```python
from build123d import *

# Parameters (mm, degrees)
SKETCH_1_R          = 14
EXTRUDE_1_DEPTH     = 4.5
CHAMFER_1_SIZE      = 2.25
SKETCH_2_R          = 10.75
EXTRUDE_2_DEPTH     = 25
CUT_EXTRUDE_START   = -25
CUT_EXTRUDE_1_DEPTH = 25
SKETCH_4_R          = 6
CUT_EXTRUDE_2_DEPTH = 5
EXTRUDE_3_DEPTH     = 5
CHAMFER_2_SIZE      = 0.5
EXTRUDE_4_DEPTH     = 3
SKETCH_7_R          = 2.5
CUT_EXTRUDE_3_DEPTH = 10


with BuildPart() as part:
    # 草图1 → 凸台-拉伸1 (new body)
    with BuildSketch(Plane(origin=(0, 0, 0), x_dir=(1, 0, 0), z_dir=(0, 1, 0))):
        with Locations(Location((0, 0, 0), (0, 0, 270))):
            Circle(SKETCH_1_R)
    extrude(amount=EXTRUDE_1_DEPTH)

    # 倒角1
    chamfer_1_edges = [part.edges().sort_by_distance(p)[0] for p in [
        (0, 4.5, -14),
    ]]
    chamfer(chamfer_1_edges, length=CHAMFER_1_SIZE)

    # 草图2 → 凸台-拉伸2 (add)
    with BuildSketch(Plane.XZ):
        with Locations(Location((0, 0, 0), (0, 0, 90))):
            Circle(SKETCH_2_R)
    extrude(amount=EXTRUDE_2_DEPTH)

    # 草图3 → 切除-拉伸1 (cut)
    with BuildSketch(Plane.XZ.offset(25).offset(CUT_EXTRUDE_START)):
        with BuildLine():
            Line((-3.94493346, -10), (3.94493346, -10))
            ThreePointArc((3.94493346, -10), (0, -10.75), (-3.94493346, -10))
        make_face()
        with BuildLine():
            Line((-3.94493346, 10), (3.94493346, 10))
            ThreePointArc((3.94493346, 10), (0, 10.75), (-3.94493346, 10))
        make_face()
    extrude(amount=CUT_EXTRUDE_1_DEPTH, mode=Mode.SUBTRACT)

    # 草图4 → 切除-拉伸2 (cut)
    with BuildSketch(Plane(origin=(0, 4.5, 0), x_dir=(1, 0, 0), z_dir=(0, 1, 0))):
        with Locations(Location((0, 0, 0), (0, 0, 270))):
            Circle(SKETCH_4_R)
    extrude(amount=-CUT_EXTRUDE_2_DEPTH, mode=Mode.SUBTRACT)

    # 草图5 → 凸台-拉伸3 (add)
    with BuildSketch(Plane(origin=(0, -0.5, 0), x_dir=(1, 0, 0), z_dir=(0, 1, 0))):
        with BuildLine():
            Line((-0.259807621, 3.05), (-2.771281292, -1.3))
            ThreePointArc((-2.771281292, -1.3), (-2.771281292, -1.6), (-2.511473671, -1.75))
            Line((-2.511473671, -1.75), (2.511473671, -1.75))
            ThreePointArc((2.511473671, -1.75), (2.771281292, -1.6), (2.771281292, -1.3))
            Line((2.771281292, -1.3), (0.259807621, 3.05))
            ThreePointArc((0.259807621, 3.05), (0, 3.2), (-0.259807621, 3.05))
        make_face()
    extrude(amount=EXTRUDE_3_DEPTH)

    # 倒角2
    chamfer_2_edges = [part.edges().sort_by_distance(p)[0] for p in [
        (0, 4.5, -6),
    ]]
    chamfer(chamfer_2_edges, length=CHAMFER_2_SIZE)

    # 草图6 → 凸台-拉伸4 (add)
    with BuildSketch(Plane.XZ.offset(25)):
        Polygon((7.071067812, 0), (0, 7.071067812), (-7.071067812, 0), (0, -7.071067812), align=None)
    extrude(amount=EXTRUDE_4_DEPTH)

    # 草图7 → 切除-拉伸3 (cut)
    with BuildSketch(Plane.XZ.offset(28)):
        with Locations(Location((0, 0, 0), (0, 0, 270))):
            Circle(SKETCH_7_R)
    extrude(amount=-CUT_EXTRUDE_3_DEPTH, mode=Mode.SUBTRACT)

    # 草图9 → 切除-旋转3 (revolve, cut)
    with BuildSketch(Plane.XY):
        Polygon((-7.071067812, -27.422649731), (-7.071067812, -28), (-6.071067812, -28), align=None)
    revolve(axis=Axis((0, 0, 0), (0, -1, 0)), mode=Mode.SUBTRACT)


solid = part.part
```
Check sheet for the modelled part. Datum: model origin and axes. Units: mm. A direction names the side the tool comes from. Give positions to 0.01 mm unless a question says otherwise; leave off trailing zeros. Write each loop counter-clockwise with the first axis right and the second up, starting at its lowest first coordinate (ties: lowest second). Pieces come first, ordered by that corner, then holes. Notation, with made-up numbers: (19.5, -9) - (78.5, -9) arc R12 ccw to (78.5, 6) - close; hole circle Ø4 at (66.25, 18). An arc over 180 degrees is marked (long way). Answer as a JSON object with one key per item and string values. Group by question number.
1) Sectioned sample at B-B (y = -12.5). Record the cut outline in (x, z).
2) Thickness scan on probe 1 along X at (y, z) = (1.95, 0); probe 2 along Y at (x, z) = (-4.5, 9); probe 3 along Y at (x, z) = (-5.25, -0.5). Record the ranges inside material, lowest first. Write a range as from..to.
3) Sectioned sample at A-A (y = -22.5). Record the cut outline in (x, z), then the cut area to 3 significant figures.
4) Release check for a two-part mould opening along Z. For faces 5 (the face through (0, -18, 0)), 6 (the face through (0.1, 0, 10.3)), 7 (the face through (3.585, -26.479, 3.486)) record: pulls with the +Z half, pulls with the -Z half, needs draft (parallel to the pull), parting line crosses it, or undercut.
5) Depth check by flat-ended pin: P1, Ø4, axis at x = 8, y = -18, coming from the +Z side; P2, Ø1.5, axis at x = -10.5, y = -10.5, coming from the +Z side; P3, Ø1, axis at x = -7.5, z = -10.5, coming from the +Y side. Enter the tip coordinate at first touch or a pass-through.
6) Access from +Z, -Z, +X, -X, +Y, -Y to the whole of each face (thin tool, end or side, straight path). Record for faces 1 (the face through (-3, -25, -5)), 2 (the face through (0, -12, 10)), 3 (the face through (-3.585, -26.479, -3.486)), 4 (the face through (0, -12, -10)).
Geometry results:
{
 "1": {"outline": "(-3.94, -10) - (3.94, -10) arc R10.75 ccw to (3.94, 10) - (-3.94, 10) arc R10.75 ccw to start"},
 "2": {"probe 1": "x = -14..-6, -2.02..2.02, 6..14", "probe 2": "y = -25..4.5", "probe 3": "y = -28..-0.5"},
 "3": {"outline": "(-3.94, -10) - (3.94, -10) arc R10.75 ccw to (3.94, 10) - (-3.94, 10) arc R10.75 ccw to start; hole circle Ø5 at (0, 0)", "area": "335 mm^2"},
 "4": {"face 5": "undercut", "face 6": "needs draft", "face 7": "pulls with the +Z half"},
 "5": {"P1": "stops at z = 8.92", "P2": "stops at z = 4.53", "P3": "stops at y = 3.85"},
 "6": {"face 1": "-Y", "face 2": "+Z, +X, -X, -Y", "face 3": "-Z, -X, -Y", "face 4": "-Z, +X, -X, -Y"}
}
